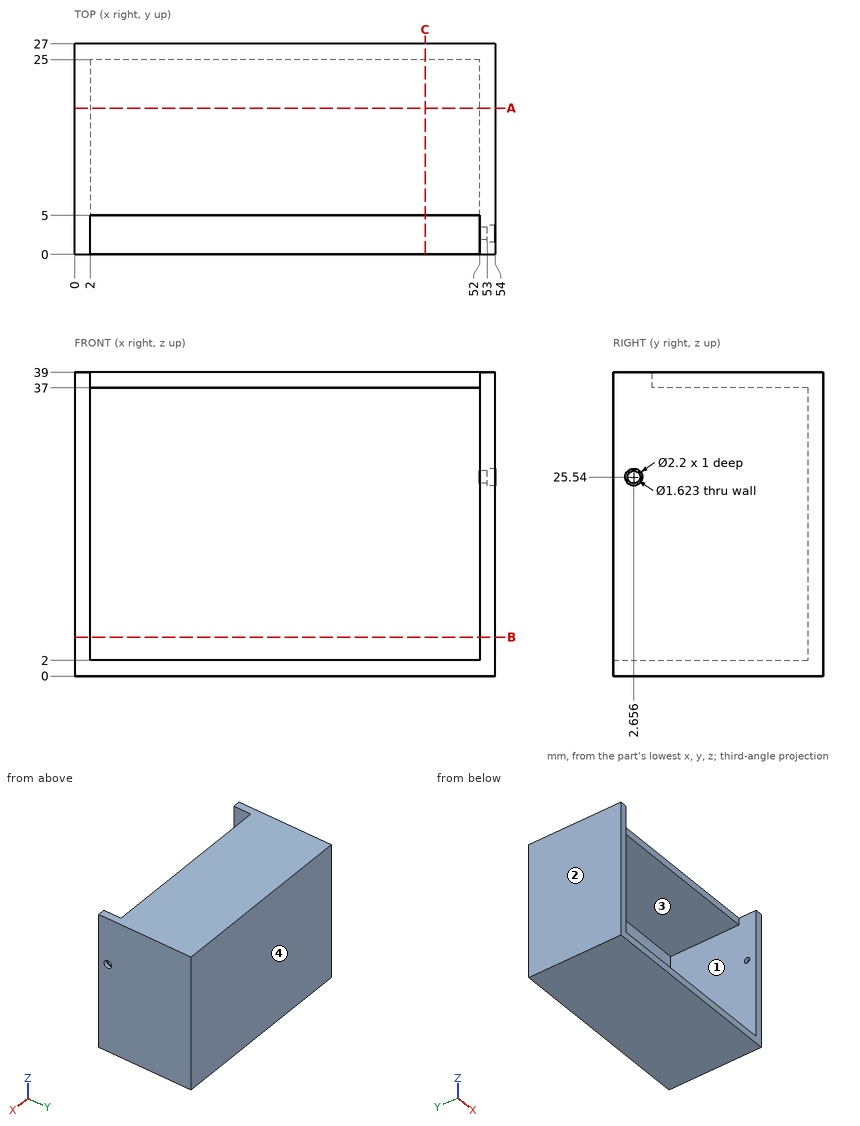
Job drawing, mm, ordinate dimensions from the low corner. One solid piece. Give positions to 0.01 mm unless a question says otherwise; leave off trailing zeros. Order: outer loops, then holes, each group sorted by start corner. A loop starts at its lowest first (then second) coordinate and runs counter-clockwise, first axis right, second up. Notation, with made-up numbers: (-6, -4) - (40, -4) arc R14 cw to (40, 20) - close; hole circle Ø7 at (57, 14). An arc over 180 degrees is marked (long way). Return JSON: item names as keys, results as strings.
1) Cut at B-B, the plane z = 5. Give the cut face in (x, y).
Geometry says:
{"outline": "(0, 0) - (2, 0) - (2, 25) - (52, 25) - (52, 0) - (54, 0) - (54, 27) - (0, 27) - close"}
2) Flat gauge pins, fed straight in: P1, Ø2, axis at x = 22.5, y = 3, coming from the -Z side; P2, Ø0.6, axis at x = 15.5, z = 38.5, coming from the -Y side; P3, Ø5, axis at x = 6, z = 6, coming from the -Y side. Where does each tip first touch, or does it go through?
Geometry says:
{"P1": "z = 0", "P2": "y = 5", "P3": "y = 25"}
3) Probe line 1 (Z direction, x = 8, y = 14); line 2 (X direction, y = 11, z = 7); line 3 (Y direction, x = 49, z = 34). List the from-to ranges inside material, lowest first. Write a range as from..to.
Geometry says:
{"line 1": "0..2, 37..39", "line 2": "0..2, 52..54", "line 3": "25..27"}
4) Cut at A-A, the plane y = 18.75. Give the cut face in (x, z).
Geometry says:
{"outline": "(0, 0) - (54, 0) - (54, 39) - (0, 39) - close; hole (2, 2) - (52, 2) - (52, 37) - (2, 37) - close"}
5) Pull direction X, two halves, no side cores. Call the marked faces 1, 2, 3 and 4: pulls with the +X half, pulls with the -X half, needs draft (parallel to the pull), parting line crosses it, or undercut.
Geometry says:
{"face 1": "undercut", "face 2": "pulls with the -X half", "face 3": "undercut", "face 4": "needs draft"}
6) Cut at C-C, the plane x = 45. Give the cut face in (y, z), plus the area to 3 significant figures.
Geometry says:
{"outline": "(0, 0) - (27, 0) - (27, 39) - (5, 39) - (5, 37) - (25, 37) - (25, 2) - (0, 2) - close", "area": "168 mm²"}
